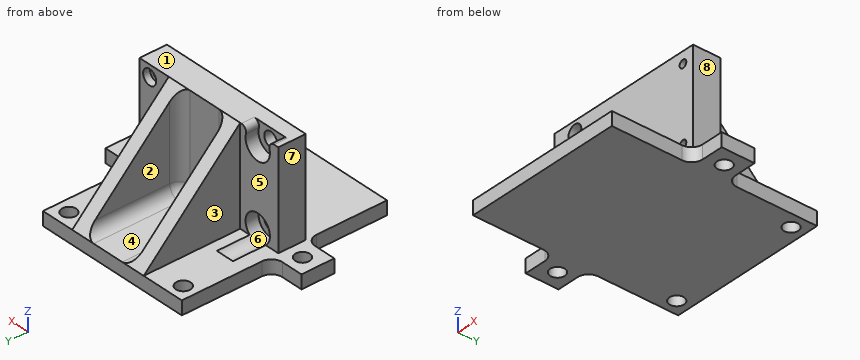
from build123d import *

# Parameters (mm, degrees)
SKETCH1_W                        = 37
SKETCH1_H                        = 22.4
BOSS_EXTRUDE1_DEPTH              = 6.35
SKETCH7_W                        = 3.175
SKETCH7_H                        = 47.610000126
BOSS_EXTRUDE2_DEPTH              = 37
CBORE_FOR_M3_SHCS3_AT_2_COUNT    = 2
CBORE_FOR_M3_SHCS3_AT_2_PITCH    = 17.5
CBORE_FOR_M1_6_SHCS1_D           = 1.8
CBORE_FOR_M1_6_SHCS1_CBORE_D     = 3.5
CBORE_FOR_M1_6_SHCS1_CBORE_DEPTH = 1.6
BOSS_EXTRUDE3_START              = -10.16
BOSS_EXTRUDE3_DEPTH              = 3.175
BOSS_EXTRUDE4_START              = -29.21
BOSS_EXTRUDE4_DEPTH              = 3.175
SKETCH18_W                       = 7.62
SKETCH18_H                       = 7.62
BOSS_EXTRUDE5_DEPTH              = 3.175
M3_CLEARANCE_HOLE1_D             = 3.4
FILLET1_R                        = 2.54
FILLET2_R                        = 1.27


with BuildPart() as part:
    # Sketch1 → Boss-Extrude1 (new body)
    with BuildSketch(Plane(origin=(0, 0, 0), x_dir=(1, 0, 0), z_dir=(0, 1, 0))):
        with Locations((18.5, 11.2)):
            Rectangle(SKETCH1_W, SKETCH1_H)
    extrude(amount=BOSS_EXTRUDE1_DEPTH)

    # Sketch7 → Boss-Extrude2 (add)
    with BuildSketch(Plane(origin=(37, 0, 0), x_dir=(0, 0, -1), z_dir=(1, 0, 0))):
        with Locations((-1.5875, 4.944999937)):
            Rectangle(SKETCH7_W, SKETCH7_H)
    extrude(amount=-BOSS_EXTRUDE2_DEPTH)

    # Sketch13 → CBORE for M3 SHCS3 (revolve, cut)
    with BuildSketch(Plane(origin=(5.5, 13.97, -2.45), x_dir=(0, 0, 1), z_dir=(1, 0, 0))):
        Polygon((0, 0), (0, 32.830000126), (1.7, 32.830000126), (1.7, 10.62), (3.25, 10.62), (3.25, 0), align=None)
    cbore_for_m3_shcs3 = revolve(axis=Axis((5.5, 20.32, -2.45), (0, -1, 0)), mode=Mode.SUBTRACT)

    # CBORE for M3 SHCS3 at 2: CBORE for M3 SHCS3 ×2
    with Locations(*[(0, 0, -i * CBORE_FOR_M3_SHCS3_AT_2_PITCH) for i in range(1, CBORE_FOR_M3_SHCS3_AT_2_COUNT)]):
        add(cbore_for_m3_shcs3, mode=Mode.SUBTRACT)

    # CBORE for M1.6 SHCS1 (through all)
    with Locations(Plane(origin=(0, 6.35, 0), x_dir=(1, 0, 0), z_dir=(0, 1, 0))):
        with Locations((34.3, 19.7), (34.3, 2.7)):
            CounterBoreHole(CBORE_FOR_M1_6_SHCS1_D / 2, CBORE_FOR_M1_6_SHCS1_CBORE_D / 2, CBORE_FOR_M1_6_SHCS1_CBORE_DEPTH)

    # Sketch16 → Boss-Extrude3 (add)
    with BuildSketch(Plane.ZY.offset(BOSS_EXTRUDE3_START)):
        Polygon((-22.4, 6.35), (0, 6.35), (0, 28.75), align=None)
    extrude(amount=-BOSS_EXTRUDE3_DEPTH)

    # Sketch16<2> → Boss-Extrude4 (add)
    with BuildSketch(Plane.ZY.offset(BOSS_EXTRUDE4_START)):
        Polygon((-22.4, 6.35), (0, 6.35), (0, 28.75), align=None)
    extrude(amount=BOSS_EXTRUDE4_DEPTH)

    # Sketch18 → Boss-Extrude5 (add, through all)
    with BuildSketch(Plane.XY):
        with Locations((40.81, 3.81)):
            Rectangle(SKETCH18_W, SKETCH18_H)
        with Locations((-3.81, 3.81)):
            Rectangle(SKETCH18_W, SKETCH18_H)
    extrude(amount=BOSS_EXTRUDE5_DEPTH)

    # M3 Clearance Hole1 (through all)
    with Locations(Plane(origin=(0, 0, 0), x_dir=(-1, 0, 0), z_dir=(0, 0, -1))):
        with Locations((-40.725, 3.985), (-33.74, 25.575), (-3.26, 25.575), (3.725, 3.985)):
            Hole(M3_CLEARANCE_HOLE1_D / 2)

    # Fillet1
    # the kernel refuses this fillet: 2.54 mm, written as the material it adds along each edge
    with BuildSketch(Plane(origin=(15.875, 8.89, -2.54), x_dir=(0, -1, 0), z_dir=(-1, 0, 0))) as fillet1_piece_1_section:
        Polygon((0, 0), (FILLET1_R, 0), (FILLET1_R, FILLET1_R), (0, FILLET1_R), align=None)
    fillet1_piece_1 = extrude(amount=FILLET1_R, mode=Mode.PRIVATE)
    fillet1_piece_1 = fillet1_piece_1 - Plane(origin=(15.875, 8.89, -2.54), x_dir=(0, 0.7071067811865475, -0.7071067811865475), z_dir=(-1, 0, 0)) * Sphere(FILLET1_R, mode=Mode.PRIVATE)
    add(fillet1_piece_1)
    with BuildSketch(Plane(origin=(23.495, 8.89, -2.54), x_dir=(1, 0, 0), z_dir=(0, -1, 0))) as fillet1_piece_2_section:
        Polygon((0, 0), (FILLET1_R, 0), (FILLET1_R, FILLET1_R), (0, FILLET1_R), align=None)
    fillet1_piece_2 = extrude(amount=FILLET1_R, mode=Mode.PRIVATE)
    fillet1_piece_2 = fillet1_piece_2 - Plane(origin=(23.495, 8.89, -2.54), x_dir=(-0.7071067811865475, 0, -0.7071067811865475), z_dir=(0, -1, 0)) * Sphere(FILLET1_R, mode=Mode.PRIVATE)
    add(fillet1_piece_2)
    with BuildSketch(Plane(origin=(0, 0, 0), x_dir=(0, -1, 0), z_dir=(0, 0, 1)), Plane(origin=(37, 7.62, 0), x_dir=(0, 1, 0), z_dir=(0, 0, 1))) as fillet1_piece_3:
        with BuildLine():
            CenterArc((FILLET1_R, -FILLET1_R), FILLET1_R, 90, 90)
            Line((0, -FILLET1_R), (0, 0))
            Line((0, 0), (FILLET1_R, 0))
        make_face()
    extrude(amount=3.175)
    with BuildSketch(Plane(origin=(0, 7.62, 0), x_dir=(0, 1, 0), z_dir=(0, 0, 1)), Plane(origin=(37, 0, 0), x_dir=(0, -1, 0), z_dir=(0, 0, 1))) as fillet1_piece_4:
        with BuildLine():
            CenterArc((FILLET1_R, FILLET1_R), FILLET1_R, 180, 90)
            Line((0, FILLET1_R), (0, 0))
            Line((0, 0), (FILLET1_R, 0))
        make_face()
    extrude(amount=3.175)
    with BuildSketch(Plane(origin=(15.875, 6.35, 0), x_dir=(0, 0, -1), z_dir=(1, 0, 0))) as fillet1_piece_5:
        with BuildLine():
            CenterArc((FILLET1_R, FILLET1_R), FILLET1_R, 180, 90)
            Line((0, FILLET1_R), (0, 0))
            Line((0, 0), (FILLET1_R, 0))
        make_face()
    extrude(amount=7.62)
    with BuildSketch(Plane(origin=(13.335, 8.89, 0), x_dir=(1, 0, 0), z_dir=(0, 1, 0))) as fillet1_piece_6_section:
        with BuildLine():
            CenterArc((FILLET1_R, FILLET1_R), FILLET1_R, 180, 90)
            Line((0, FILLET1_R), (0, 0))
            Line((0, 0), (FILLET1_R, 0))
        make_face()
    fillet1_piece_6 = extrude(amount=19.86, mode=Mode.PRIVATE)
    fillet1_piece_6 = split(fillet1_piece_6, bisect_by=Plane(origin=(13.919159385, 23.364808453, -5.385191547), z_dir=(0, -0.7071067811865476, 0.7071067811865476)), keep=Keep.TOP, mode=Mode.PRIVATE)
    add(fillet1_piece_6)
    with BuildSketch(Plane(origin=(13.335, 6.35, -22.4), x_dir=(1, 0, 0), z_dir=(0, 0, 1))) as fillet1_piece_7_section:
        with BuildLine():
            CenterArc((FILLET1_R, FILLET1_R), FILLET1_R, 180, 90)
            Line((0, FILLET1_R), (0, 0))
            Line((0, 0), (FILLET1_R, 0))
        make_face()
    fillet1_piece_7 = extrude(amount=19.86, mode=Mode.PRIVATE)
    fillet1_piece_7 = split(fillet1_piece_7, bisect_by=Plane(origin=(13.919159385, 11.735191547, -17.014808453), z_dir=(0, -0.7071067811865476, 0.7071067811865476)), keep=Keep.TOP, mode=Mode.PRIVATE)
    add(fillet1_piece_7)
    with BuildSketch(Plane(origin=(26.035, 6.35, -22.4), x_dir=(-1, 0, 0), z_dir=(0, 0, 1))) as fillet1_piece_8_section:
        with BuildLine():
            CenterArc((FILLET1_R, -FILLET1_R), FILLET1_R, 90, 90)
            Line((0, -FILLET1_R), (0, 0))
            Line((0, 0), (FILLET1_R, 0))
        make_face()
    fillet1_piece_8 = extrude(amount=19.86, mode=Mode.PRIVATE)
    fillet1_piece_8 = split(fillet1_piece_8, bisect_by=Plane(origin=(25.450840615, 11.735191547, -17.014808453), z_dir=(0, -0.7071067811865476, 0.7071067811865476)), keep=Keep.TOP, mode=Mode.PRIVATE)
    add(fillet1_piece_8)
    with BuildSketch(Plane(origin=(26.035, 8.89, 0), x_dir=(-1, 0, 0), z_dir=(0, 1, 0))) as fillet1_piece_9_section:
        with BuildLine():
            CenterArc((FILLET1_R, -FILLET1_R), FILLET1_R, 90, 90)
            Line((0, -FILLET1_R), (0, 0))
            Line((0, 0), (FILLET1_R, 0))
        make_face()
    fillet1_piece_9 = extrude(amount=19.86, mode=Mode.PRIVATE)
    fillet1_piece_9 = split(fillet1_piece_9, bisect_by=Plane(origin=(25.450840615, 23.364808453, -5.385191547), z_dir=(0, -0.7071067811865476, 0.7071067811865476)), keep=Keep.TOP, mode=Mode.PRIVATE)
    add(fillet1_piece_9)

    # Fillet2
    fillet2_edges = [part.edges().sort_by_distance(p)[0] for p in [
        (7.63541565, 4.85, -22.4),
        (3.36458435, 4.85, -22.4),
    ]]
    fillet(fillet2_edges, radius=FILLET2_R)


with BuildPart() as body_2:
    # Mirror1: mirrored copy
    add(part.part.mirror(Plane.XY))


solid = body_2.part
Could you check a few things on this model? Use its own coordinates, in mm. Face numbers are marked on the shaded views. A direction names the side the tool comes from. Give positions to 0.01 mm unless a question says otherwise; leave off trailing zeros. Write each loop counter-clockwise with the first axis right and the second up, starting at its lowest first coordinate (ties: lowest second). Pieces come first, ordered by that corner, then holes. Notation, with made-up numbers: (33.25, 31) -> (79.25, 31) arc R31 ccw to (79.25, 59) -> close; hole circle Ø1 at (51.25, -17.5). An arc over 180 degrees is marked (long way). Write each question's results on one line, items separated by ' | '. Start each with the question number.
Q1. Suppose I cut it at C-C, the plane y = -9. List the corners of the cut face in (x, z) for me (3 decimals).
Q2. Suppose I cut it at A-A, the plane y = 20. List the corners of the cut face in (x, z) for me (3 decimals).
Q3. Which directions (+Z, -Z, +X, -X, +Y, -Y) give clear straight access to the entire face, cutting with the end or side of a thin tool? Please do the marked faces 4, 5, 6, 7 and 8.
Q4. Suppose I cut it at B-B, the plane x = 34.3. List the corners of the cut face in (y, z) for me (3 decimals).
Q5. I need wall thicknesses on probe 1 along Z at (x, y) = (5.5, 2.45) (3 decimals); probe 2 along Z at (x, y) = (34.3, 5.45) (3 decimals); probe 3 along X at (y, z) = (15, 5.5) (3 decimals). Which ranges of each line are inside material? Lowest first, please.
Q6. I'm going to push flat-ended pins straight in: pin 1 Ø4 at (x, y) = (33.74, 25.575) entering from +Z; pin 2 Ø8.5 at (y, z) = (13.5, 7) entering from +X; pin 3 Ø3 at (x, z) = (27, 16.5) entering from +Y. Where does each tip first touch, or does it pass through?
Q7. We'd pull the mould along X, two halves only. Please class the marked faces 1, 2 and 3: +X half, -X half, draft (parallel to the pull), parting line (faces both ways), or undercut.
Outcome:
1) outline: (0, -3.175) -> (37, -3.175) -> (37, 0) -> (0, 0) -> close
2) outline: (0, -3.175) -> (37, -3.175) -> (37, 0) -> (29.21, 0) -> (29.21, 8.75) -> (26.035, 8.75) -> (26.035, 2.54) arc R2.54 cw to (23.495, 0) -> (15.875, 0) arc R2.54 cw to (13.335, 2.54) -> (13.335, 8.75) -> (10.16, 8.75) -> (10.16, 0) -> (0, 0) -> close
3) face 4: +Z, +Y | face 5: +Z, -X, +Y | face 6: none | face 7: +Z, -X, +Y, -Y | face 8: +Z, +X, +Y, -Y
4) outline: (-18.86, -3.175) -> (23.97, -3.175) -> (23.97, 0) -> (6.35, 0) -> (6.35, 0.95) -> (4.75, 0.95) -> (4.75, 1.8) -> (0, 1.8) -> (0, 0) -> (-18.86, 0) -> close; (0, 3.6) -> (4.75, 3.6) -> (4.75, 4.45) -> (6.35, 4.45) -> (6.35, 17.95) -> (4.75, 17.95) -> (4.75, 18.8) -> (0, 18.8) -> close; (0, 20.6) -> (4.75, 20.6) -> (4.75, 21.45) -> (6.35, 21.45) -> (6.35, 22.4) -> (0, 22.4) -> close; (27.18, -3.175) -> (28.75, -3.175) -> (28.75, 0) -> (27.18, 0) -> close
5) probe 1: -3.175 to 0.75, 4.15 to 18.25, 21.65 to 22.4 | probe 2: -3.175 to 0.95, 4.45 to 17.95, 21.45 to 22.4 | probe 3: 10.16 to 13.335, 26.035 to 29.21
6) pin 1: z = 0 | pin 2: x = 29.21 | pin 3: y = 13.75
7) face 1: draft | face 2: undercut | face 3: -X half
